from build123d import *

# Parameters (mm, degrees)
SKETCH1_R           = 10.65
SKETCH1_R_2         = 8.65
BOSS_EXTRUDE1_DEPTH = 227
SKETCH2_R           = 3.5
CUT_EXTRUDE1_DEPTH  = 228.499109888
LPATTERN1_COUNT     = 2
LPATTERN1_PITCH     = 150


with BuildPart() as part:
    # Sketch1 → Boss-Extrude1 (new body)
    with BuildSketch(Plane.XY):
        with Locations(Location((0, 0, 0), (0, 0, 180))):
            Circle(SKETCH1_R)
        with Locations(Location((0, 0, 0), (0, 0, 180))):
            Circle(SKETCH1_R_2, mode=Mode.SUBTRACT)
    extrude(amount=BOSS_EXTRUDE1_DEPTH)

    # Sketch2 → Cut-Extrude1 (cut, symmetric)
    with BuildSketch(Plane(origin=(0, 0, 0), x_dir=(1, 0, 0), z_dir=(0, 1, 0))):
        with Locations(Location((0, -177, 0), (0, 0, 270))):
            Circle(SKETCH2_R)
    cut_extrude1 = extrude(amount=CUT_EXTRUDE1_DEPTH, both=True, mode=Mode.SUBTRACT)

    # LPattern1: Cut-Extrude1 ×2
    with Locations(*[(0, 0, -i * LPATTERN1_PITCH) for i in range(1, LPATTERN1_COUNT)]):
        add(cut_extrude1, mode=Mode.SUBTRACT)


solid = part.part
Could you check a few things on this model? Use its own coordinates, in mm. Give positions to 0.01 mm unless a question says otherwise; leave off trailing zeros. Write each loop counter-clockwise with the first axis right and the second up, starting at its lowest first coordinate (ties: lowest second). Pieces come first, ordered by that corner, then holes. Notation, with made-up numbers: (19, 53) -> (71, 53) arc R18 ccw to (71, 66) -> close; hole circle Ø5 at (88, -10). An arc over 180 degrees is marked (long way). Write each question's results on one line, items separated by ' | '. Start each with the question number.
Q1. Suppose I cut it at A-A, the plane x = 0. List the corners of the cut face in (y, z) for me, and give its area (3 significant figures).
Q2. We'd pull the mould along Z, two halves only. Please class faces 1 (the face through (0, -9, 227)), 2 (the face through (-10.158, -3.199, 111.911)), 3 (the face through (1.05, -9.26, 30.34)): +Z half, -Z half, draft (parallel to the pull), parting line (faces both ways), or undercut.
Q3. I'm going to push flat-ended pins straight in: pin 1 Ø6 at (y, z) = (-5, 177.5) entering from -X; pin 2 Ø1 at (y, z) = (4.5, 114.5) entering from -X; pin 3 Ø3 at (y, z) = (-5, 84) entering from -X. Where does each tip first touch, or does it pass through?
Q4. Suppose I cut it at C-C, the plane z = 177. List the corners of the cut face in (x, y) for me, and give its area (3 significant figures).
Q5. Suppose I cut it at B-B, the plane y = 3. List the corners of the cut face in (x, z) for me, and give its area (3 significant figures).
Q6. Suppose I cut it at D-D, the plane z = 122.5. List the corners of the cut face in (x, y) for me.
Q7. I need wall thicknesses on probe 1 along Z at (x, y) = (0, -9.6); probe 2 along Y at (x, z) = (-2, 149); probe 3 along Y at (x, z) = (4, 78). Which ranges of each line are inside material? Lowest first, please.
Outcome:
1) outline: (-10.65, 0) -> (-8.65, 0) -> (-8.65, 23.5) -> (-10.65, 23.5) -> close; (-10.65, 30.5) -> (-8.65, 30.5) -> (-8.65, 173.5) -> (-10.65, 173.5) -> close; (-10.65, 180.5) -> (-8.65, 180.5) -> (-8.65, 227) -> (-10.65, 227) -> close; (8.65, 0) -> (10.65, 0) -> (10.65, 23.5) -> (8.65, 23.5) -> close; (8.65, 30.5) -> (10.65, 30.5) -> (10.65, 173.5) -> (8.65, 173.5) -> close; (8.65, 180.5) -> (10.65, 180.5) -> (10.65, 227) -> (8.65, 227) -> close | area: 852 mm2
2) face 1: +Z half | face 2: draft | face 3: undercut
3) pin 1: x = -10.46 | pin 2: x = -9.87 | pin 3: x = -10.06
4) outline: (-3.5, -10.06) -> (-3.5, -7.91) arc R8.65 cw to (-3.5, 7.91) -> (-3.5, 10.06) arc R10.65 ccw to start; (3.5, -10.06) arc R10.65 ccw to (3.5, 10.06) -> (3.5, 7.91) arc R8.65 cw to (3.5, -7.91) -> close | area: 92.6 mm2
5) outline: (-10.22, 0) -> (-8.11, 0) -> (-8.11, 227) -> (-10.22, 227) -> close; (8.11, 0) -> (10.22, 0) -> (10.22, 227) -> (8.11, 227) -> close | area: 956 mm2
6) outline: circle Ø21.3 at (0, 0); hole circle Ø17.3 at (0, 0)
7) probe 1: 0 to 23.5, 30.5 to 173.5, 180.5 to 227 | probe 2: -10.46 to -8.42, 8.42 to 10.46 | probe 3: -9.87 to -7.67, 7.67 to 9.87
